Model file for the job. Use its own axes, mm. Coordinates: 2 decimals unless noted, no trailing zeros. Loops run counter-clockwise (first coordinate to the right, second up) from the corner with the lowest first, then second, coordinate; pieces in that order, holes last. Notation, with made-up numbers: (-31.5, 79.25) - (23.5, 79.25) arc R14 ccw to (23.5, 87.25) - close; hole circle Ø4 at (48, 41.25). An arc over 180 degrees is marked (long way). Write each question's results on one line, items separated by ' | '. Start each with the question number.
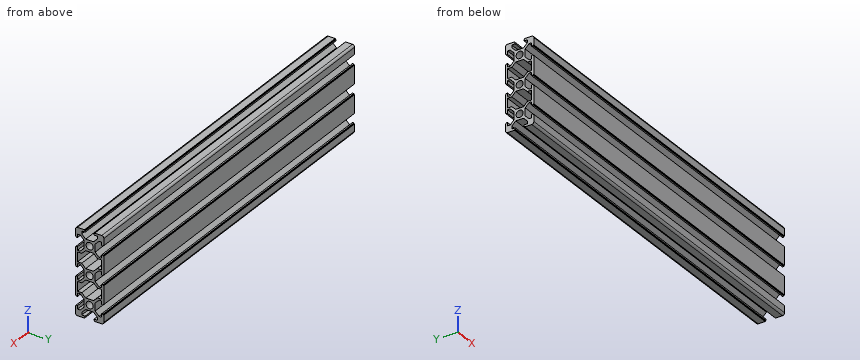
```python
from build123d import *

# Parameters (mm, degrees)
SKETCH1_R                = 2.5
F_20_X_20_X_R1_5_1_DEPTH = 265


with BuildPart() as part:
    # Sketch1 → 铝型材 20 X 20 X R1.5(1) (new body)
    with BuildSketch(Plane(origin=(548.637296324, 8.985389246, 0), x_dir=(0, 1, 0), z_dir=(1, 0, 0))):
        with BuildLine():
            Line((-10, -3.6), (-9.5, -3.6))
            Line((-9.5, -3.6), (-9.5, -3.1))
            Line((-9.5, -3.1), (-8.5, -3.1))
            Line((-8.5, -3.1), (-8.5, -5.5))
            Line((-8.5, -5.5), (-6.65, -5.5))
            Line((-6.65, -5.5), (-3.9, -2.75))
            Line((-3.9, -2.75), (-3.9, 2.75))
            Line((-3.9, 2.75), (-6.65, 5.5))
            Line((-6.65, 5.5), (-8.5, 5.5))
            Line((-8.5, 5.5), (-8.5, 3.1))
            Line((-8.5, 3.1), (-9.5, 3.1))
            Line((-9.5, 3.1), (-9.5, 3.6))
            Line((-9.5, 3.6), (-10, 3.6))
            Line((-10, 3.6), (-10, 8.5))
            Line((-10, 8.5), (-10, 11.5))
            Line((-10, 11.5), (-10, 16.4))
            Line((-10, 16.4), (-9.5, 16.4))
            Line((-9.5, 16.4), (-9.5, 16.9))
            Line((-9.5, 16.9), (-8.5, 16.9))
            Line((-8.5, 16.9), (-8.5, 14.5))
            Line((-8.5, 14.5), (-6.65, 14.5))
            Line((-6.65, 14.5), (-3.9, 17.25))
            Line((-3.9, 17.25), (-3.9, 22.75))
            Line((-3.9, 22.75), (-6.65, 25.5))
            Line((-6.65, 25.5), (-8.5, 25.5))
            Line((-8.5, 25.5), (-8.5, 23.1))
            Line((-8.5, 23.1), (-9.5, 23.1))
            Line((-9.5, 23.1), (-9.5, 23.6))
            Line((-9.5, 23.6), (-10, 23.6))
            Line((-10, 23.6), (-10, 28.5))
            Line((-10, 28.5), (-10, 31.5))
            Line((-10, 31.5), (-10, 36.4))
            Line((-10, 36.4), (-9.5, 36.4))
            Line((-9.5, 36.4), (-9.5, 36.9))
            Line((-9.5, 36.9), (-8.5, 36.9))
            Line((-8.5, 36.9), (-8.5, 34.5))
            Line((-8.5, 34.5), (-6.65, 34.5))
            Line((-6.65, 34.5), (-3.9, 37.25))
            Line((-3.9, 37.25), (-3.9, 42.75))
            Line((-3.9, 42.75), (-6.65, 45.5))
            Line((-6.65, 45.5), (-8.5, 45.5))
            Line((-8.5, 45.5), (-8.5, 43.1))
            Line((-8.5, 43.1), (-9.5, 43.1))
            Line((-9.5, 43.1), (-9.5, 43.6))
            Line((-9.5, 43.6), (-10, 43.6))
            Line((-10, 43.6), (-10, 48.5))
            ThreePointArc((-10, 48.5), (-9.560660172, 49.560660172), (-8.5, 50))
            Line((-8.5, 50), (-3.6, 50))
            Line((-3.6, 50), (-3.6, 49.5))
            Line((-3.6, 49.5), (-3.1, 49.5))
            Line((-3.1, 49.5), (-3.1, 48.5))
            Line((-3.1, 48.5), (-5.5, 48.5))
            Line((-5.5, 48.5), (-5.5, 46.65))
            Line((-5.5, 46.65), (-2.75, 43.9))
            Line((-2.75, 43.9), (2.75, 43.9))
            Line((2.75, 43.9), (5.5, 46.65))
            Line((5.5, 46.65), (5.5, 48.5))
            Line((5.5, 48.5), (3.1, 48.5))
            Line((3.1, 48.5), (3.1, 49.5))
            Line((3.1, 49.5), (3.6, 49.5))
            Line((3.6, 49.5), (3.6, 50))
            Line((3.6, 50), (8.5, 50))
            ThreePointArc((8.5, 50), (9.560660172, 49.560660172), (10, 48.5))
            Line((10, 48.5), (10, 43.6))
            Line((10, 43.6), (9.5, 43.6))
            Line((9.5, 43.6), (9.5, 43.1))
            Line((9.5, 43.1), (8.5, 43.1))
            Line((8.5, 43.1), (8.5, 45.5))
            Line((8.5, 45.5), (6.65, 45.5))
            Line((6.65, 45.5), (3.9, 42.75))
            Line((3.9, 42.75), (3.9, 37.25))
            Line((3.9, 37.25), (6.65, 34.5))
            Line((6.65, 34.5), (8.5, 34.5))
            Line((8.5, 34.5), (8.5, 36.9))
            Line((8.5, 36.9), (9.5, 36.9))
            Line((9.5, 36.9), (9.5, 36.4))
            Line((9.5, 36.4), (10, 36.4))
            Line((10, 36.4), (10, 31.5))
            Line((10, 31.5), (10, 28.5))
            Line((10, 28.5), (10, 23.6))
            Line((10, 23.6), (9.5, 23.6))
            Line((9.5, 23.6), (9.5, 23.1))
            Line((9.5, 23.1), (8.5, 23.1))
            Line((8.5, 23.1), (8.5, 25.5))
            Line((8.5, 25.5), (6.65, 25.5))
            Line((6.65, 25.5), (3.9, 22.75))
            Line((3.9, 22.75), (3.9, 17.25))
            Line((3.9, 17.25), (6.65, 14.5))
            Line((6.65, 14.5), (8.5, 14.5))
            Line((8.5, 14.5), (8.5, 16.9))
            Line((8.5, 16.9), (9.5, 16.9))
            Line((9.5, 16.9), (9.5, 16.4))
            Line((9.5, 16.4), (10, 16.4))
            Line((10, 16.4), (10, 11.5))
            Line((10, 11.5), (10, 8.5))
            Line((10, 8.5), (10, 3.6))
            Line((10, 3.6), (9.5, 3.6))
            Line((9.5, 3.6), (9.5, 3.1))
            Line((9.5, 3.1), (8.5, 3.1))
            Line((8.5, 3.1), (8.5, 5.5))
            Line((8.5, 5.5), (6.65, 5.5))
            Line((6.65, 5.5), (3.9, 2.75))
            Line((3.9, 2.75), (3.9, -2.75))
            Line((3.9, -2.75), (6.65, -5.5))
            Line((6.65, -5.5), (8.5, -5.5))
            Line((8.5, -5.5), (8.5, -3.1))
            Line((8.5, -3.1), (9.5, -3.1))
            Line((9.5, -3.1), (9.5, -3.6))
            Line((9.5, -3.6), (10, -3.6))
            Line((10, -3.6), (10, -8.5))
            ThreePointArc((10, -8.5), (9.560660172, -9.560660172), (8.5, -10))
            Line((8.5, -10), (3.6, -10))
            Line((3.6, -10), (3.6, -9.5))
            Line((3.6, -9.5), (3.1, -9.5))
            Line((3.1, -9.5), (3.1, -8.5))
            Line((3.1, -8.5), (5.5, -8.5))
            Line((5.5, -8.5), (5.5, -6.65))
            Line((5.5, -6.65), (2.75, -3.9))
            Line((2.75, -3.9), (-2.75, -3.9))
            Line((-2.75, -3.9), (-5.5, -6.65))
            Line((-5.5, -6.65), (-5.5, -8.5))
            Line((-5.5, -8.5), (-3.1, -8.5))
            Line((-3.1, -8.5), (-3.1, -9.5))
            Line((-3.1, -9.5), (-3.6, -9.5))
            Line((-3.6, -9.5), (-3.6, -10))
            Line((-3.6, -10), (-8.5, -10))
            ThreePointArc((-8.5, -10), (-9.560660172, -9.560660172), (-10, -8.5))
            Line((-10, -8.5), (-10, -3.6))
        make_face()
        Circle(SKETCH1_R, mode=Mode.SUBTRACT)
        with Locations((0, 20)):
            Circle(SKETCH1_R, mode=Mode.SUBTRACT)
        with Locations((0, 40)):
            Circle(SKETCH1_R, mode=Mode.SUBTRACT)
        Polygon((-5.5, 6.65), (-8.5, 6.65), (-8.5, 13.35), (-5.5, 13.35), (-2.75, 16.1), (2.75, 16.1), (5.5, 13.35), (8.5, 13.35), (8.5, 6.65), (5.5, 6.65), (2.75, 3.9), (-2.75, 3.9), align=None, mode=Mode.SUBTRACT)
        Polygon((-5.5, 26.65), (-8.5, 26.65), (-8.5, 33.35), (-5.5, 33.35), (-2.75, 36.1), (2.75, 36.1), (5.5, 33.35), (8.5, 33.35), (8.5, 26.65), (5.5, 26.65), (2.75, 23.9), (-2.75, 23.9), align=None, mode=Mode.SUBTRACT)
    extrude(amount=F_20_X_20_X_R1_5_1_DEPTH)


solid = part.part
```
Q1. Cut at C-C (z = 11). List the corners of the cut face in (x, y).
Q2. Cut at A-A (z = 0). List the corners of the cut face in (x, y), and give its area (3 significant figures).
Q3. Drill centre lines: L1, parallel to Z at x = 731, y = 1; L2, parallel to Y at x = 787.5, z = 32.5; L3, parallel to Z at x = 640, y = 8. Where is each one in solid material? Low to high. Write a range as from..to.
Q4. Pin check, flat tips, straight feed: pin 1 (2 mm diameter, centred on x = 782.5, z = -1.5, fed in from +Y); pin 2 (0.6 mm diameter, centred on x = 664.5, y = -0.5, fed in from -Z); pin 3 (5 mm diameter, centred on x = 750.5, y = 9.5, fed in from -Z). Stop position of each tip, or through.
Q5. Cut at B-B (x = 605.5). State how many separate pieces and enclosed holes the cut face has, and give its area (3 significant figures).
Check result:
1) outline: (548.64, -1.01) - (813.64, -1.01) - (813.64, 0.49) - (548.64, 0.49) - close; (548.64, 17.49) - (813.64, 17.49) - (813.64, 18.99) - (548.64, 18.99) - close
2) outline: (548.64, 5.09) - (813.64, 5.09) - (813.64, 6.49) - (548.64, 6.49) - close; (548.64, 11.49) - (813.64, 11.49) - (813.64, 12.89) - (548.64, 12.89) - close | area: 742 mm²
3) L1: -10..-5.5, 5.5..6.65, 13.35..14.5, 25.5..26.65, 33.35..34.5, 45.5..50 | L2: -1.01..0.49, 17.49..18.99 | L3: -3.9..-2.3, 2.3..3.9, 16.1..17.7, 22.3..23.9, 36.1..37.7, 42.3..43.9
4) pin 1: y = 12.89 | pin 2: z = -9.83 | pin 3: z = -4.16
5) separate pieces: 1 | enclosed holes: 5 | area: 398 mm²
